Can you work these out from the model? Positions are in its coordinate system, mm. Round coordinates to 2 decimals unless told otherwise and drop trailing zeros. Write each loop counter-clockwise with the first axis right and the second up, starting at its lowest first coordinate (ties: lowest second). Pieces come first, ordered by that corner, then holes. Notation, with made-up numbers: M 0.5,67 L 57.5,67 A38 ccw 57.5,106 Z; hole C 65,22.5 d2. An arc over 180 degrees is marked long. Answer in a Markdown table with one row per item. Add a question column.
(1) If I drill on probe 1 along X at (y, z) = (1.5, -46.99); probe 2 along X at (y, z) = (0.75, -3.81); probe 3 along X at (y, z) = (0.7, -43), over which ranges is the centre line in solid material (lowest first)?
(2) Suppose I cut it at B-B, the plane x = 48. Write out the boundary of the cut face in (y, z).
(3) Suppose I cut it at A-A, the plane y = 0.5. Write out the boundary of the cut face in (x, z).
(4) I'm going to push a flat-ended pin straight in: pin 1 (1 mm diameter, centred on x = 46, y = 0.5, fed in from -Z). Where does the tip first touch, or does it pass through?
from build123d import *

# Parameters (mm, degrees)
SKETCH_1_R      = 1.5
EXTRUDE_1_DEPTH = 2
FILLET_1_R      = 3


with BuildPart() as part:
    # 草图1 → 凸台-拉伸1 (new body)
    with BuildSketch(Plane(origin=(0, 0, 0), x_dir=(1, 0, 0), z_dir=(0, 1, 0))):
        Polygon((0, 0), (96.27, 0), (96.27, 50.8), (59.18, 50.8), (59.18, 38.48), (37.08, 38.48), (37.08, 50.8), (0, 50.8), align=None)
        with Locations(Location((20.063894942, 46.982706601, 0), (0, 0, 270))):
            Circle(SKETCH_1_R, mode=Mode.SUBTRACT)
        with Locations(Location((76.193894468, 46.99, 0), (0, 0, 90))):
            Circle(SKETCH_1_R, mode=Mode.SUBTRACT)
        with Locations(Location((76.193894468, 3.81, 0), (0, 0, 270))):
            Circle(SKETCH_1_R, mode=Mode.SUBTRACT)
        with Locations(Location((20.063894942, 3.817293399, 0), (0, 0, 270))):
            Circle(SKETCH_1_R, mode=Mode.SUBTRACT)
    extrude(amount=EXTRUDE_1_DEPTH)

    # 圆角1
    fillet_1_edges = [part.edges().sort_by_distance(p)[0] for p in [
        (37.08, 1, -50.8),
        (37.08, 1, -38.48),
        (59.18, 1, -38.48),
        (59.18, 1, -50.8),
        (96.27, 1, -50.8),
        (96.27, 1, 0),
        (0, 1, 0),
        (0, 1, -50.8),
    ]]
    fillet(fillet_1_edges, radius=FILLET_1_R)


solid = part.part
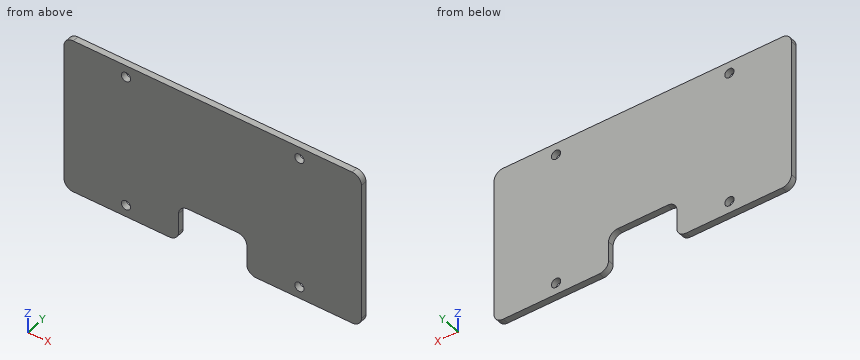
Calculated:
| question | item | result |
|---|---|---|
| 1 | probe 1 | 0 to 18.56, 21.56 to 37.08, 59.18 to 74.69, 77.69 to 96.27 |
| 1 | probe 2 | 0 to 18.56, 21.56 to 74.69, 77.69 to 96.27 |
| 1 | probe 3 | 0 to 37.08, 59.18 to 96.27 |
| 2 | outline | M 0,-38.48 L 2,-38.48 L 2,0 L 0,0 Z |
| 3 | outline | M 0,-47.8 A3 ccw 3,-50.8 L 34.08,-50.8 A3 ccw 37.08,-47.8 L 37.08,-41.48 A3 cw 40.08,-38.48 L 56.18,-38.48 A3 cw 59.18,-41.48 L 59.18,-47.8 A3 ccw 62.18,-50.8 L 93.27,-50.8 A3 ccw 96.27,-47.8 L 96.27,-3 A3 ccw 93.27,0 L 3,0 A3 ccw 0,-3 Z; hole C 20.06,-46.98 d3; hole C 20.06,-3.82 d3; hole C 76.19,-46.99 d3; hole C 76.19,-3.81 d3 |
| 4 | pin 1 | z = -38.48 |
